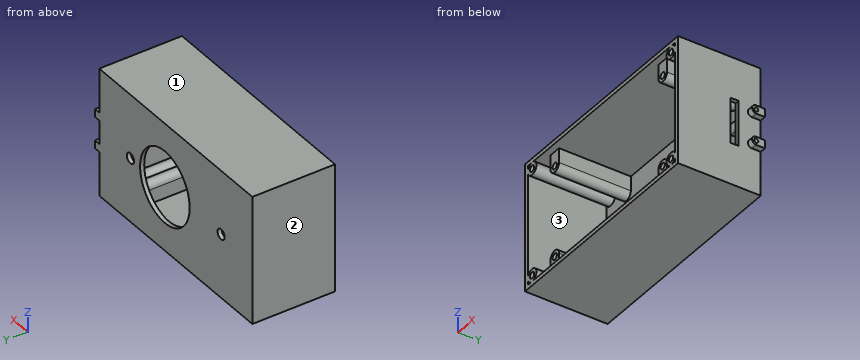
```python
from build123d import *

# Parameters (mm, degrees)
F0_W           = 108
F0_H           = 62
F1_DEPTH       = 40
F2_W           = 104
F2_H           = 58
F3_DEPTH       = 38
F5_START       = -3.25
F5_DEPTH       = 34.75
F6_R           = 3.05
F7_DEPTH       = 38
F8_R           = 1.5
F9_DEPTH       = 15
F10_R          = 1.5
F11_DEPTH      = 18.5
F12_R          = 17.5
F12_R_2        = 2.5
F13_DEPTH      = 40.001
F16_DEPTH      = 15
F16_DEPTH_BACK = 3
F17_W          = 4
F17_H          = 22
F18_DEPTH      = 2
F19_R          = 1
F20_DEPTH      = 10
F20_DEPTH_BACK = 5


with BuildPart() as f1:
    # F0 (on Front) → F1 (new body)
    with BuildSketch(Plane.XZ):
        Rectangle(F0_W, F0_H)
    extrude(amount=-F1_DEPTH)

    # F2 (on Front) → F3 (cut)
    with BuildSketch(Plane.XZ):
        Rectangle(F2_W, F2_H)
    extrude(amount=-F3_DEPTH, mode=Mode.SUBTRACT)

    # F4 (on Front) → F5 (join)
    with BuildSketch(Plane.XZ.offset(F5_START)):
        with BuildLine():
            ThreePointArc((-40.73, 22), (-37.73, 19), (-34.73, 22))
            ThreePointArc((-34.73, 22), (-37.73, 25), (-40.73, 22))
        make_face()
        with BuildLine():
            ThreePointArc((-40.73, 22), (-37.73, 25), (-34.73, 22))
            Line((-34.73, 22), (-34.73, 29.0249657466))
            Line((-34.73, 29.0249657466), (-40.73, 29.0249657466))
            Line((-40.73, 29.0249657466), (-40.73, 22))
        make_face()
        with BuildLine():
            ThreePointArc((35.45, 22), (38.45, 19), (41.45, 22))
            ThreePointArc((41.45, 22), (38.45, 25), (35.45, 22))
        make_face()
        with BuildLine():
            ThreePointArc((35.45, 22), (38.45, 25), (41.45, 22))
            Line((41.45, 22), (41.45, 29.0909428149))
            Line((41.45, 29.0909428149), (35.45, 29.1012134403))
            Line((35.45, 29.1012134403), (35.45, 22))
        make_face()
        with BuildLine():
            ThreePointArc((-40.73, -22.2), (-37.73, -25.2), (-34.73, -22.2))
            ThreePointArc((-34.73, -22.2), (-37.73, -19.2), (-40.73, -22.2))
        make_face()
        with BuildLine():
            Line((-34.73, -29.2853660554), (-34.73, -22.2))
            ThreePointArc((-34.73, -22.2), (-37.73, -25.2), (-40.73, -22.2))
            Line((-40.73, -22.2), (-40.73, -29.2745608509))
            Line((-40.73, -29.2745608509), (-34.73, -29.2853660554))
        make_face()
        with BuildLine():
            ThreePointArc((35.45, -22.2), (38.45, -25.2), (41.45, -22.2))
            ThreePointArc((41.45, -22.2), (38.45, -19.2), (35.45, -22.2))
        make_face()
        with BuildLine():
            Line((41.45, -29.2963500738), (41.45, -22.2))
            ThreePointArc((41.45, -22.2), (38.45, -25.2), (35.45, -22.2))
            Line((35.45, -22.2), (35.45, -29.2963500738))
            Line((35.45, -29.2963500738), (41.45, -29.2963500738))
        make_face()
    extrude(amount=-F5_DEPTH)

    # F6 (on Front) → F7 (join, through all)
    with BuildSketch(Plane.XZ):
        with Locations((-49, 26)):
            Circle(F6_R)
        with Locations((49, 26)):
            Circle(F6_R)
        with Locations((49, -26)):
            Circle(F6_R)
        with Locations((-49, -26)):
            Circle(F6_R)
    extrude(amount=-F7_DEPTH)

    # F8 (on Front) → F9 (cut)
    with BuildSketch(Plane.XZ):
        with Locations((-49, 26)):
            Circle(F8_R)
        with Locations((-49, -26)):
            Circle(F8_R)
        with Locations((49, -26)):
            Circle(F8_R)
        with Locations((49, 26)):
            Circle(F8_R)
    extrude(amount=-F9_DEPTH, mode=Mode.SUBTRACT)

    # F10 (on Front) → F11 (cut)
    with BuildSketch(Plane.XZ):
        with Locations((-37.73, 22)):
            Circle(F10_R)
        with Locations((-37.73, -22.2)):
            Circle(F10_R)
        with Locations((38.45, 22)):
            Circle(F10_R)
        with Locations((38.45, -22.2)):
            Circle(F10_R)
    extrude(amount=-F11_DEPTH, mode=Mode.SUBTRACT)

    # F12 (on Front) → F13 (cut, through all)
    with BuildSketch(Plane.XZ):
        with Locations((7.7104928971, 0)):
            Circle(F12_R)
        with Locations((-32, 0)):
            Circle(F12_R_2)
        with Locations((32, 0)):
            Circle(F12_R_2)
    extrude(amount=-F13_DEPTH, mode=Mode.SUBTRACT)

    # F15 (on offset) → F16 (join, two sides)
    with BuildSketch(Plane.YZ.offset(54)) as f16_sk:
        with BuildLine():
            Line((40, 9.5658428478), (35.7879940012, 9.6248040744))
            ThreePointArc((35.7879940012, 9.6248040744), (33.7602591267, 7.5928062172), (35.8523524108, 5.6271333798))
            Line((35.8523524108, 5.6271333798), (40, 5.6271333798))
            Line((40, 5.6271333798), (40, 9.5658428478))
        make_face()
        with BuildLine():
            Line((40, -5.7445825184), (35.8167641743, -5.6258057052))
            ThreePointArc((35.8167641743, -5.6258057052), (33.7602698715, -7.5921455752), (35.7510600226, -9.6249800191))
            ThreePointArc((35.7510600226, -9.6249800191), (35.76, -9.625), (35.7689399774, -9.6249800191))
            Line((35.7689399774, -9.6249800191), (40, -9.6249800191))
            Line((40, -9.6249800191), (40, -5.7445825184))
        make_face()
    extrude(amount=-F16_DEPTH)
    extrude(f16_sk.sketch, amount=F16_DEPTH_BACK)

    # F17 (on offset) → F18 (cut, through all)
    with BuildSketch(Plane.YZ.offset(54)):
        with Locations((27.26, 0)):
            Rectangle(F17_W, F17_H)
    extrude(amount=-F18_DEPTH, mode=Mode.SUBTRACT)

    # F19 (on offset) → F20 (cut, two sides)
    with BuildSketch(Plane.YZ.offset(54)) as f20_sk:
        with Locations((35.76, 7.625)):
            Circle(F19_R)
        with Locations((35.76, -7.625)):
            Circle(F19_R)
    extrude(amount=-F20_DEPTH, mode=Mode.SUBTRACT)
    extrude(f20_sk.sketch, amount=F20_DEPTH_BACK, mode=Mode.SUBTRACT)


solid = f1.part
```
Can you work these out from the model? Positions are in its coordinate system, mm. Face numbers are marked on the shaded views. Coordinates: 2 decimals unless noted, no trailing zeros. Loops run counter-clockwise (first coordinate to the right, second up) from the corner with the lowest first, then second, coordinate; pieces in that order, holes last.
1) Imagine slicing it at D-D on y = 30.5. State how many separate pieces and enclosed holes the cut face has, plus the area to 3 significant figures.
2) I need wall thicknesses on probe 1 along Z at (x, y) = (3.5, 12.5); probe 2 along Z at (x, y) = (38.5, 23); probe 3 along X at (y, z) = (31, -21.5). Which ranges of each line are inside material? Lowest first, please.
3) For pin 1 (6 mm diameter, centred on x = 42, z = 9.5, fed in from -Y); pin 2 (1.5 mm diameter, centred on x = -38, z = -23, fed in from -Y); pin 3 (1.8 mm diameter, centred on x = -49, z = -26, fed in from -Y), each with a flat end and sliding along its axis, tell me the tip position at first contact or that it passes through.
4) Imagine slicing it at A-A on z = 0. List the corners of the cut face in (x, y) for me.
5) Imagine slicing it at C-C on x = -37.73. List the corners of the cut face in (y, z) for me.
6) Imagine slicing it at B-B on x = 2. List the corners of the cut face in (y, z) for me, plus the area to 3 significant figures.
7) Thinking about a two-plate mould opening in Z: for the marked faces 1, 2 and 3, which applies, pulls with the +Z half, pulls with the -Z half, needs draft (parallel to the pull), parting line crosses it, or undercut?
Completed:
1. separate pieces: 1
1. enclosed holes: 5
1. area: 1,000 mm2
2. probe 1: z = -31 to -29, 29 to 31
2. probe 2: z = -31 to -19.2, 19 to 31
2. probe 3: x = -54 to -52, -40.65 to -34.81, 35.53 to 41.37, 52 to 54
3. pin 1: stops at y = 33.76
3. pin 2: stops at y = 3.25
3. pin 3: stops at y = 15
4. outline: (-54, 0) - (-52, 0) - (-52, 38) - (-34.5, 38) - (-34.5, 40) - (-54, 40) - close; (-29.5, 38) - (-9.79, 38) - (-9.79, 40) - (-29.5, 40) - close; (25.21, 38) - (29.5, 38) - (29.5, 40) - (25.21, 40) - close; (34.5, 38) - (52, 38) - (52, 29.26) - (54, 29.26) - (54, 40) - (34.5, 40) - close; (52, 0) - (54, 0) - (54, 25.26) - (52, 25.26) - close
5. outline: (0, -31) - (40, -31) - (40, 31) - (0, 31) - (0, 29) - (3.25, 29) - (3.25, 23.5) - (18.5, 23.5) - (18.5, 20.5) - (3.25, 20.5) - (3.25, 19) - (38, 19) - (38, -19.2) - (3.25, -19.2) - (3.25, -20.7) - (18.5, -20.7) - (18.5, -23.7) - (3.25, -23.7) - (3.25, -29) - (0, -29) - close
6. outline: (0, -31) - (40, -31) - (40, -16.54) - (38, -16.54) - (38, -29) - (0, -29) - close; (0, 29) - (38, 29) - (38, 16.54) - (40, 16.54) - (40, 31) - (0, 31) - close
6. area: 210 mm2
7. face 1: pulls with the +Z half
7. face 2: needs draft
7. face 3: undercut
